from build123d import *

# Parameters (mm, degrees)
F1_DEPTH = 50.8
F2_W     = 141.4932012558
F2_H     = 197.677500546
F3_DEPTH = 25.4
F4_R     = 1.5875
F5_DEPTH = 25.4
F6_R     = 2.38125
F7_DEPTH = 25.4
F8_R     = 5.08


with BuildPart() as f1:
    # F0 (on Right) → F1 (new body, symmetric)
    with BuildSketch(Plane.YZ):
        Polygon((-9.8313118777, -5.1045094135), (-73.3876270169, -5.1045094135), (-73.3876270169, -5.8665094135), (-9.8313118777, -5.8665094135), (40.9123729831, -5.8665094135), (40.9123729831, -5.1045094135), align=None)
    extrude(amount=F1_DEPTH, both=True)

    # F2 (on Top) → F3 (cut)
    with BuildSketch(Plane.XY):
        with Locations((-0.8716285229, -40.7481454313)):
            Rectangle(F2_W, F2_H)
        with BuildLine():
            Line((-13.740606685, -65.7309788432), (-20.0346057486, 17.8250920772))
            ThreePointArc((-20.0346057486, 17.8250920772), (2.1903942514, 40.9123729831), (24.4153942514, 17.8250920772))
            Line((24.4153942514, 17.8250920772), (21.184393315, -67.0376270169))
            Line((21.184393315, -67.0376270169), (14.834393315, -73.3876270169))
            Line((14.834393315, -73.3876270169), (-13.740606685, -65.7309788432))
        make_face(mode=Mode.SUBTRACT)
    extrude(amount=-F3_DEPTH, mode=Mode.SUBTRACT)

    # F4 (on face) → F5 (cut)
    with BuildSketch(Plane.XY.offset(-5.1045094135)):
        with Locations((-10.0768637425, -60.1386720603)):
            Circle(F4_R)
        with Locations((2.1903942514, -63.4256739331)):
            Circle(F4_R)
        with Locations((14.4576522453, -66.7126758059)):
            Circle(F4_R)
    extrude(amount=-F5_DEPTH, mode=Mode.SUBTRACT)

    # F6 (on face) → F7 (cut)
    with BuildSketch(Plane.XY.offset(-5.1045094135)):
        with Locations((1.1186605513, 34.5623729831)):
            Circle(F6_R)
    extrude(amount=-F7_DEPTH, mode=Mode.SUBTRACT)

    # F8
    f8_edges = [f1.edges().sort_by_distance(p)[0] for p in [
        (-13.740607, -65.730979, -5.485509),
        (14.834393, -73.387627, -5.485509),
        (21.184393, -67.037627, -5.485509),
    ]]
    fillet(f8_edges, radius=F8_R)


solid = f1.part
Design review of the part built by this model. Coordinates are the model's own, in mm. Give positions to 0.01 mm unless a question says otherwise; leave off trailing zeros. Order: outer loops, then holes, each group sorted by start corner. A loop starts at its lowest first (then second) coordinate and runs counter-clockwise, first axis right, second up.
1. Mouldability with a two-part tool opening along Y and no side actions: class faces 1 (the flat face through (3, -15, -5.105)), 2 (the cylindrical face through (-10.284, -58.565, -5.48)), 3 (the flat face through (-16.98, -22.72, -5.48)) as +Y half, -Y half, draft (parallel to the pull), parting line (faces both ways), or undercut.
Solution:
face 1: draft
face 2: undercut
face 3: -Y half
2. Add section B-B, the plane y = 26. State the section outline as (x, z) points, then the cut area to 3 significant figures.
Solution:
outline: (-18.81, -5.87) - (23.19, -5.87) - (23.19, -5.1) - (-18.81, -5.1) - close
area: 32.0 mm2
3. Add section A-A, the plane z = -5.5. State the section outline as (x, y) points (1 decimal).
Solution:
outline: (-20, 17.8) - (-14, -62.1) arc R5.1 ccw to (-10.3, -66.7) - (12, -72.6) arc R5.1 ccw to (16.9, -71.3) - (19.8, -68.4) arc R5.1 ccw to (21.3, -65) - (24.4, 17.8) arc R22.2 ccw (long way) to start; hole circle Ø3.2 at (-10.1, -60.1); hole circle Ø4.8 at (1.1, 34.6); hole circle Ø3.2 at (2.2, -63.4); hole circle Ø3.2 at (14.5, -66.7)
4. To check wall thickness, follow L1, parallel to Y at x = 3, z = -5.8; L2, parallel to Y at x = 0.5, z = -5.2; L3, parallel to X at y = -65.5, z = -5.2. State the ranges of each line that lie inside material, in increasing order.
Solution:
L1: y = -70.22 to -64.79, -62.06 to 33.1, 36.02 to 40.9
L2: y = -69.55 to 32.26, 36.86 to 40.85
L3: x = -12.38 to 13.43, 15.48 to 21.22
5. Add section C-C, the plane x = -6.5. State the section outline as (y, z) points, then the cut area to 3 significant figures.
Solution:
outline: (-67.67, -5.87) - (39.14, -5.87) - (39.14, -5.1) - (-67.67, -5.1) - close
area: 81.4 mm2
